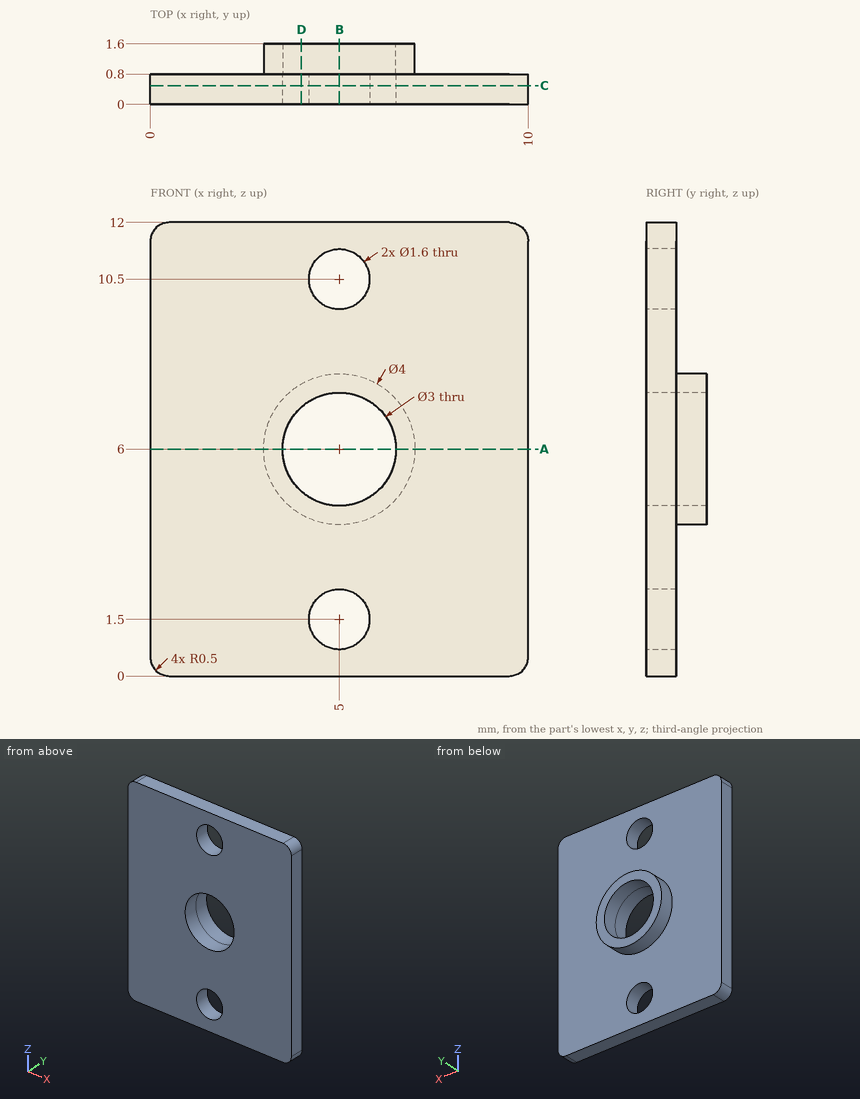
Design review of the part shown in the three views and the two pictorial views. Dimensions are in mm from the part's minimum x, y and z. Round coordinates to 2 decimals unless told otherwise and drop trailing zeros. Write each loop counter-clockwise with the first axis right and the second up, starting at its lowest first coordinate (ties: lowest second). Pieces come first, ordered by that corner, then holes.
Item 1: Clearance check with flat-ended pins moving along their axes: pin 1 Ø1.8 at (x, z) = (5, 6) entering from -Y; pin 2 Ø1 at (x, z) = (7, 10) entering from +Y. State where each tip first meets the part, or that it passes through.
Item 2: We need section C-C on y = 0.5. Write out the cut boundary in (x, z), and give its area (3 significant figures).
Item 3: We need section D-D on x = 4. Write out the cut boundary in (y, z).
Item 4: We need section B-B on x = 5. Write out the cut boundary in (y, z).
Item 5: We need section A-A on z = 6. Write out the cut boundary in (x, y), and give its area (3 significant figures).
Item 6: For probe 1 along Z at (x, y) = (5, 0.65); probe 2 along X at (y, z) = (0.2, 6); probe 3 along X at (y, z) = (1.4, 6), list the stretches that pass through material, from the lowest coordinate up.
Returned:
1. pin 1: passes through
1. pin 2: stops at y = 0.8
2. outline: (0, 0.5) arc R0.5 ccw to (0.5, 0) - (9.5, 0) arc R0.5 ccw to (10, 0.5) - (10, 11.5) arc R0.5 ccw to (9.5, 12) - (0.5, 12) arc R0.5 ccw to (0, 11.5) - close; hole circle Ø3 at (5, 6); hole circle Ø1.6 at (5, 1.5); hole circle Ø1.6 at (5, 10.5)
2. area: 109 mm2
3. outline: (0, 0) - (0.8, 0) - (0.8, 4.27) - (1.6, 4.27) - (1.6, 4.88) - (0, 4.88) - close; (0, 7.12) - (1.6, 7.12) - (1.6, 7.73) - (0.8, 7.73) - (0.8, 12) - (0, 12) - close
4. outline: (0, 0) - (0.8, 0) - (0.8, 0.7) - (0, 0.7) - close; (0, 2.3) - (0.8, 2.3) - (0.8, 4) - (1.6, 4) - (1.6, 4.5) - (0, 4.5) - close; (0, 7.5) - (1.6, 7.5) - (1.6, 8) - (0.8, 8) - (0.8, 9.7) - (0, 9.7) - close; (0, 11.3) - (0.8, 11.3) - (0.8, 12) - (0, 12) - close
5. outline: (0, 0) - (3.5, 0) - (3.5, 1.6) - (3, 1.6) - (3, 0.8) - (0, 0.8) - close; (6.5, 0) - (10, 0) - (10, 0.8) - (7, 0.8) - (7, 1.6) - (6.5, 1.6) - close
5. area: 6.40 mm2
6. probe 1: z = 0 to 0.7, 2.3 to 4.5, 7.5 to 9.7, 11.3 to 12
6. probe 2: x = 0 to 3.5, 6.5 to 10
6. probe 3: x = 3 to 3.5, 6.5 to 7
